Here's the drawing with two shaded views (mm, measured from the low corner). I have some questions. A direction names the side the tool comes from. Coordinates: 2 decimals unless noted, no trailing zeros. Order: outer loops, then holes, each group sorted by start corner. A loop starts at its lowest first (then second) coordinate and runs counter-clockwise, first axis right, second up. Notation, with made-up numbers: (78, -1.75) - (121, -1.75) arc R8 ccw to (121, 2.25) - close; hole circle Ø2 at (36.25, 33). An arc over 180 degrees is marked (long way). Answer as CSV lines item,"result". Start each with the question number.
1. I want a section at B-B, the plane x = 14.5. List the corners of the cut face in (y, z) for me.
2. I need wall thicknesses on probe 1 along X at (y, z) = (7.5, 9); probe 2 along X at (y, z) = (11.75, 10.5); probe 3 along X at (y, z) = (7.5, 5.25). Which ranges of each line are inside material? Lowest first, please.
3. Thinking about a two-plate mould opening in Y: for the marked faces 3, 4 and 5, which applies, released by +Y, released by -Y, zero draft, split by the parting line, or undercut?
4. I want a section at D-D, the plane y = 2.5. List the corners of the cut face in (x, z) for me, and give its area (3 significant figures).
5. For the marked faces 1 and 2, which set-ups out of +Z, -Z, +X, -X, +Y, -Y let a thin tool reach every point of the face, with its end or its side?
6. I want a section at A-A, the plane z = 9.25. List the corners of the cut face in (x, y) for me.
7. For pin 1 (3.5 mm diameter, centred on x = 14.5, y = 7.5, fed in from +Z), with a flat end and sliding along its axis, tell me the tip position at first contact or that it passes through.
8. I want a section at C-C, the plane y = 7.5. List the corners of the cut face in (x, z) for me, and give its area (3 significant figures).
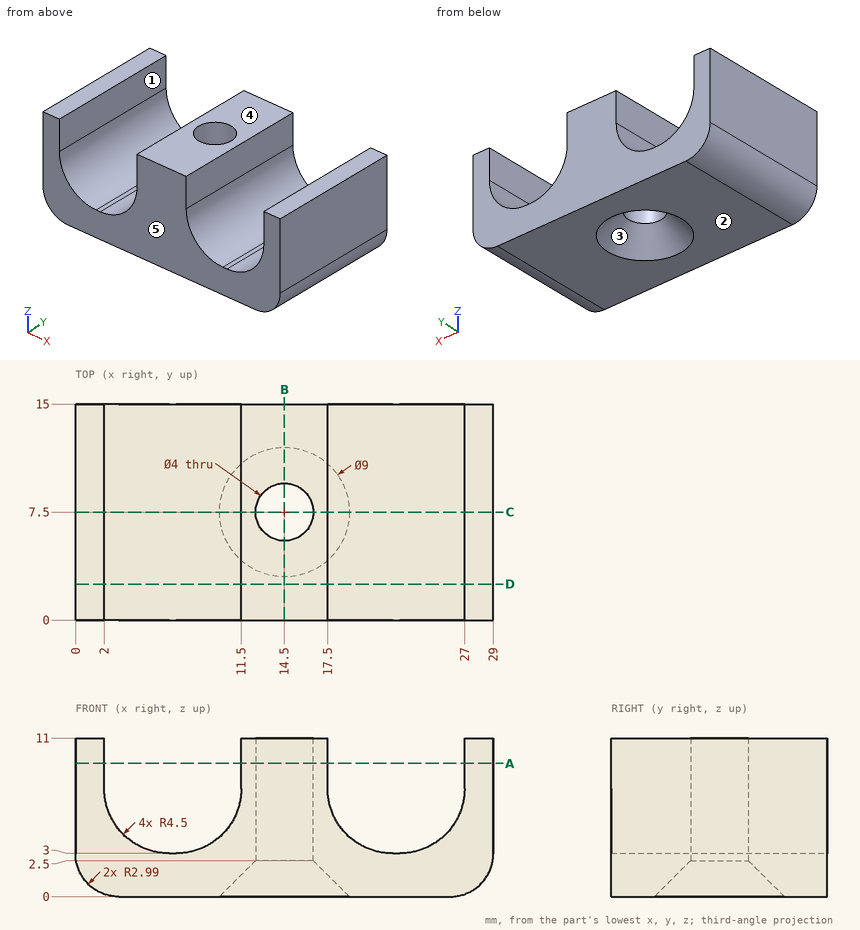
Solved:
1,outline,"(0, 0) - (3, 0) - (5.5, 2.5) - (5.5, 11) - (0, 11) - close; (9.5, 2.5) - (12, 0) - (15, 0) - (15, 11) - (9.5, 11) - close"
2,probe 1,"x = 0 to 2, 11.5 to 12.5, 16.5 to 17.5, 27 to 29"
2,probe 2,"x = 0 to 2, 11.5 to 17.5, 27 to 29"
2,probe 3,"x = 0 to 2.6, 10.9 to 12.5, 16.5 to 18.1, 26.4 to 29"
3,face 3,"undercut"
3,face 4,"zero draft"
3,face 5,"released by -Y"
4,outline,"(0, 2.99) arc R2.99 ccw to (2.99, 0) - (26.01, 0) arc R2.99 ccw to (29, 2.99) - (29, 11) - (27, 11) - (27, 7.5) arc R4.5 cw to (22.5, 3) - (22, 3) arc R4.5 cw to (17.5, 7.5) - (17.5, 11) - (11.5, 11) - (11.5, 7.5) arc R4.5 cw to (7, 3) - (6.5, 3) arc R4.5 cw to (2, 7.5) - (2, 11) - (0, 11) - close"
4,area,"181 mm2"
5,face 1,"+Z, +Y, -Y"
5,face 2,"-Z, +X, -X, +Y, -Y"
6,outline,"(0, 0) - (2, 0) - (2, 15) - (0, 15) - close; (11.5, 0) - (17.5, 0) - (17.5, 15) - (11.5, 15) - close; (27, 0) - (29, 0) - (29, 15) - (27, 15) - close; hole circle Ø4 at (14.5, 7.5)"
7,pin 1,"passes through"
8,outline,"(0, 2.99) arc R2.99 ccw to (2.99, 0) - (10, 0) - (12.5, 2.5) - (12.5, 11) - (11.5, 11) - (11.5, 7.5) arc R4.5 cw to (7, 3) - (6.5, 3) arc R4.5 cw to (2, 7.5) - (2, 11) - (0, 11) - close; (16.5, 2.5) - (19, 0) - (26.01, 0) arc R2.99 ccw to (29, 2.99) - (29, 11) - (27, 11) - (27, 7.5) arc R4.5 cw to (22.5, 3) - (22, 3) arc R4.5 cw to (17.5, 7.5) - (17.5, 11) - (16.5, 11) - close"
8,area,"130 mm2"
